```python
from build123d import *

# Parameters (mm, degrees)
F1_DEPTH = 63.5
F2_DEPTH = 7.9375
F0_W     = 25.4
F0_H     = 19.05
F3_DEPTH = 25.4
F5_R     = 6.35


with BuildPart() as f1:
    # F0 (on Front) → F1 (new body, symmetric)
    with BuildSketch(Plane.XZ):
        Polygon((41.275, -9.525), (41.275, 9.525), (22.225, 9.525), (-41.275, 9.525), (-41.275, -9.525), align=None)
    extrude(amount=F1_DEPTH, both=True)

    # F0 (on Front) → F2 (join, symmetric)
    with BuildSketch(Plane.XZ):
        with BuildLine():
            Line((-41.275, 9.525), (22.225, 9.525))
            Line((22.225, 9.525), (22.225, 27.0002))
            ThreePointArc((22.225, 27.0002), (31.5771327037, 50.7864162449), (54.6249475016, 61.8338006591))
            add(Edge.make_bspline(
                [(-41.275, 9.525), (-41.5838216247, 41.7459421201), (18.5290584876, 60.1514932336), (54.6249475016, 61.8338006591)],
                knots=[0, 0, 0, 0, 108.9228268403, 108.9228268403, 108.9228268403, 108.9228268403], degree=3))
        make_face()
    extrude(amount=F2_DEPTH, both=True)

    # F0 (on Front) → F3 (join, symmetric)
    with BuildSketch(Plane.XZ):
        with BuildLine():
            Line((22.225, 9.525), (41.275, 9.525))
            Line((41.275, 9.525), (41.275, 27.0002))
            ThreePointArc((41.275, 27.0002), (45.9246798487, 38.2255201513), (57.15, 42.8752))
            Line((57.15, 42.8752), (60.325, 42.8752))
            Line((60.325, 42.8752), (60.325, 61.9252))
            Line((60.325, 61.9252), (57.15, 61.9252))
            add(Edge.make_bspline(
                [(54.6249475016, 61.8338006591), (55.4804990504, 61.8736750261), (56.3225580044, 61.9041543798), (57.15, 61.9252)],
                knots=[108.9228268403, 108.9228268403, 108.9228268403, 108.9228268403, 111.5045361635, 111.5045361635, 111.5045361635, 111.5045361635], degree=3))
            ThreePointArc((54.6249475016, 61.8338006591), (31.5771327037, 50.7864162449), (22.225, 27.0002))
            Line((22.225, 27.0002), (22.225, 9.525))
        make_face()
        with Locations((73.025, 52.4002)):
            Rectangle(F0_W, F0_H)
    extrude(amount=F3_DEPTH, both=True)

    # F0 (on Front) → F4 (revolve)
    with BuildSketch(Plane.XZ):
        Polygon((85.725, 61.9252), (85.725, 42.8752), (85.725, 38.1), (111.125, 38.1), (111.125, 66.675), (85.725, 66.675), align=None)
    revolve(axis=Axis((85.725, 0, 52.3875), (0, 0, -1)))

    # F5
    f5_edges = [f1.edges().sort_by_distance(p)[0] for p in [
        (41.275, -63.5, 0),
        (-41.275, -63.5, 0),
        (41.275, 63.5, 0),
        (-41.275, 63.5, 0),
    ]]
    fillet(f5_edges, radius=F5_R)


solid = f1.part
```
CAD build for the part. Positions are in the model's coordinates, mm. A direction names the side the tool comes from. Coordinates: 2 decimals unless noted, no trailing zeros. Write each loop counter-clockwise with the first axis right and the second up, starting at its lowest first coordinate (ties: lowest second). Pieces come first, ordered by that corner, then holes.
(1) Two-plate mould, pull along X, no slides. Class faces 1 (the face through (-39.464, 61.59, -0.133)), 2 (the face through (-1, -1, -9.525)), 3 (the face through (60, 2, 42.875)): +X half, -X half, draft (parallel to the pull), parting line (faces both ways), or undercut.
(2) Flat gauge pins, fed straight in: pin 1 (5 mm diameter, centred on y = 18, z = 18, fed in from -X) (3 decimals); pin 2 (16.5 mm diameter, centred on x = -16, y = 40.5, fed in from +Z) (3 decimals); pin 3 (12 mm diameter, centred on x = -5, z = 14, fed in from +Y); pin 4 (12 mm diameter, centred on y = 11.5, z = 4.5, fed in from +X) (3 decimals). Where does each tip first touch, or does it go through?
(3) 3-axis set-ups, long thin cutter, end or side, ignore diameter. For faces 4 (the face through (46, -25.4, 42)), 5 (the face through (31.828, 16.547, 51.053)), 6 (the face through (86, 0, 38.1)), 7 (the face through (60, -2, 61.925)): which of +Z, -Z, +X, -X, +Y, -Y reach the whole face in a straight line?
(4) Cut at B-B, the plane y = 31. List the corners of the cut face in (x, z) (3 decimals).
(5) Drill centre lines: probe 1 along Y at (x, z) = (-22.5, 16); probe 2 along Z at (x, y) = (-8, 38) (3 decimals); probe 3 along X at (y, z) = (10, -0.5) (3 decimals). Where is each one in solid material? Low to high.
(6) Cut at A-A, the plane z = -2. List the corners of the cut face in (x, y) (3 decimals), and give its area (3 significant figures).
Geometry says:
1. face 1: -X half
1. face 2: draft
1. face 3: undercut
2. pin 1: stops at x = 22.225
2. pin 2: stops at z = 9.525
2. pin 3: stops at y = 63.5
2. pin 4: stops at x = 41.275
3. face 4: +Z, +X, -X, -Y
3. face 5: +Z, -X, +Y
3. face 6: -Z, +X, +Y, -Y
3. face 7: +Z, -X
4. outline: (-41.275, -9.525) - (41.275, -9.525) - (41.275, 9.525) - (-41.275, 9.525) - close
5. probe 1: y = -7.94 to 7.94
5. probe 2: z = -9.525 to 9.525
5. probe 3: x = -41.275 to 41.275
6. outline: (-41.275, -57.15) arc R6.35 ccw to (-34.925, -63.5) - (34.925, -63.5) arc R6.35 ccw to (41.275, -57.15) - (41.275, 57.15) arc R6.35 ccw to (34.925, 63.5) - (-34.925, 63.5) arc R6.35 ccw to (-41.275, 57.15) - close
6. area: 10,400 mm2
